Geometry check sheet. Reference: the model listing, model coordinates, mm. A direction names the side the tool comes from. Give positions to 0.01 mm unless a question says otherwise; leave off trailing zeros. Order: outer loops, then holes, each group sorted by start corner. A loop starts at its lowest first (then second) coordinate and runs counter-clockwise, first axis right, second up. Notation, with made-up numbers: M 55,11.5 L 105,11.5 A14 ccw 105,15.5 Z; hole C -4.5,53.5 d5. An arc over 180 degrees is marked long. Answer as CSV lines item,"result".
from build123d import *

# Parameters (mm, degrees)
SALIENTE_EXTRUIR1_DEPTH = 3


with BuildPart() as part:
    # Model → Saliente-Extruir1 (new body)
    with BuildSketch(Plane.XY):
        with BuildLine():
            Line((9.740547774, -46.101668317), (9.740547774, -31.803295278))
            ThreePointArc((9.740547774, -31.803295278), (9.736055246, -31.708612265), (9.722618028, -31.614779984))
            ThreePointArc((9.722618028, -31.614779984), (9.661571414, -30.916777437), (9.743772485, -30.220948989))
            ThreePointArc((9.743772485, -30.220948989), (10.255649641, -29.553355931), (11.095913023, -29.512659959))
            ThreePointArc((11.095913023, -29.512659959), (12.483349153, -29.956983983), (13.921978985, -30.186651266))
            ThreePointArc((13.921978985, -30.186651266), (14.934379735, -29.557617963), (14.625590492, -28.406406697))
            ThreePointArc((14.625590492, -28.406406697), (13.477036488, -27.648728099), (12.214507774, -27.101668317))
            ThreePointArc((12.214507774, -27.101668317), (13.791868666, -27.302020525), (15.363211574, -27.058936478))
            ThreePointArc((15.363211574, -27.058936478), (16.074009796, -26.101668317), (15.363211574, -25.144400157))
            ThreePointArc((15.363211574, -25.144400157), (14.062919208, -24.911447806), (12.743919539, -24.984021259))
            ThreePointArc((12.743919539, -24.984021259), (13.929279153, -24.357532563), (14.796143037, -23.334736147))
            ThreePointArc((14.796143037, -23.334736147), (14.817045797, -22.393544381), (14.0469262, -21.852069843))
            ThreePointArc((14.0469262, -21.852069843), (11.511931096, -22.017503021), (9.214507774, -23.101668317))
            ThreePointArc((9.214507774, -23.101668317), (4.080372041, -24.629353346), (1.714507774, -29.435168317))
            Line((1.714507774, -29.435168317), (1.714507774, -46.101668317))
            Line((1.714507774, -46.101668317), (9.740547774, -46.101668317))
        make_face()
    extrude(amount=SALIENTE_EXTRUIR1_DEPTH)


solid = part.part
(1) Tool access check on faces 1 (the face through (14.823, -22.406, 1.479)), 2 (the face through (9.741, -39, 1)), 3 (the face through (12.46, -29.95, 1.48)). Record the directions out of +Z, -Z, +X, -X, +Y, -Y that give a thin tool (end or side, any length) a straight path to the whole face; none if there is none.
The answers:
face 1,"+Z, -Z, +X"
face 2,"+Z, -Z, +X, -Y"
face 3,"+Z, -Z, -Y"
(2) Section check B-B on x = 13.5. Enter the section's corners in (y, z).
The answers:
outline,"M -30.14,0 L -27.66,0 L -27.66,3 L -30.14,3 Z; M -27.3,0 L -24.9,0 L -24.9,3 L -27.3,3 Z; M -24.65,0 L -21.81,0 L -21.81,3 L -24.65,3 Z"
(3) Section check C-C on y = -40.25. Enter the section's corners in (x, z).
The answers:
outline,"M 1.71,0 L 9.74,0 L 9.74,3 L 1.71,3 Z"
(4) Section check D-D on x = 2.5. Enter the section's corners in (y, z).
The answers:
outline,"M -46.1,0 L -26.58,0 L -26.58,3 L -46.1,3 Z"
(5) Material ranges on line 1 (X direction, y = -40, z = 1.65); line 2 (Y direction, x = 9, z = 2.85); line 3 (Y direction, x = 3.5, z = 1.9), recorded low to high.
The answers:
line 1,"x = 1.71 to 9.74"
line 2,"y = -46.1 to -23.08"
line 3,"y = -46.1 to -25.18"
(6) Draft check along Y on faces 4 (the face through (14.93, -29.57, 1.48)), 5 (the face through (16.074, -26.12, 1.479)), 6 (the face through (7, -34, 3)), 7 (the face through (13.8, -27.3, 1.5)). Enter one of: +Y half, -Y half, draft (parallel to the pull), parting line (faces both ways), or undercut.
The answers:
face 4,"undercut"
face 5,"parting line"
face 6,"draft"
face 7,"undercut"
(7) Section check A-A on z = 0.65. Enter the section's corners in (x, y).
The answers:
outline,"M 1.71,-46.1 L 9.74,-46.1 L 9.74,-31.8 A1 ccw 9.72,-31.61 A3.43 cw 9.74,-30.22 A1 cw 11.1,-29.51 A9.62 ccw 13.92,-30.19 A1 ccw 14.63,-28.41 A7.91 ccw 12.21,-27.1 A5.7 ccw 15.36,-27.06 A1 ccw 15.36,-25.14 A5.7 ccw 12.74,-24.98 A3.54 ccw 14.8,-23.33 A1 ccw 14.05,-21.85 A6.8 ccw 9.21,-23.1 A6.69 ccw 1.71,-29.44 Z"
(8) Gauge pin test, flat ends, axial feed: P1, Ø1.5, axis at y = -36, z = 0.5, coming from the +X side; P2, Ø5, axis at x = 3.5, y = -39, coming from the -Z side; P3, Ø1.5, axis at x = 6, z = 1, coming from the +Y side. Record the tip position at first contact, or that the pin passes through.
The answers:
P1,"stops at x = 9.74"
P2,"stops at z = 0"
P3,"stops at y = -23.26"
